CAD build for the part. Positions are in the model's coordinates, mm. A direction names the side the tool comes from. Coordinates: 2 decimals unless noted, no trailing zeros. Loops run counter-clockwise (first coordinate to the right, second up) from the corner with the lowest first, then second, coordinate; pieces in that order, holes last. Notation, with made-up numbers: (-33.75, -33) -> (22.25, -33) arc R13 cw to (22.25, -13) -> close; hole circle Ø1 at (-24, 9). An arc over 180 degrees is marked (long way). Answer as CSV lines item,"result". Start each with the question number.
```python
from build123d import *

# Parameters (mm, degrees)
SKETCH1_W               = 22.75
SKETCH1_H               = 11.15
BOSS_EXTRUDE1_DEPTH     = 19.5
SKETCH2_W               = 29.8
SKETCH2_H               = 13.8
SKETCH2_W_2             = 20.9
SKETCH2_H_2             = 8.8
BOSS_EXTRUDE2_DEPTH     = 2
FILLET1_R               = 1
BOSS_EXTRUDE3_DEPTH     = 4.5
FILLET2_R               = 1
SKETCH4_W               = 0.8
SKETCH4_H               = 6.4
BOSS_EXTRUDE4_DEPTH     = 8.7
CHAMFER1_SIZE           = 1
SKETCH5_W               = 29
SKETCH5_H               = 6.5
BOSS_EXTRUDE5_DEPTH     = 8.7
SKETCH6_W               = 22.75
SKETCH6_H               = 11.78
BOSS_EXTRUDE6_DEPTH     = 3.5
CHAMFER2_SIZE           = 0.5
CUT_EXTRUDE1_DEPTH      = 34.821116013
CUT_EXTRUDE1_DEPTH_BACK = 34.821116013
SKETCH7_R               = 0.871711707


with BuildPart() as part:
    # Sketch1 → Boss-Extrude1 (new body)
    with BuildSketch(Plane(origin=(0, 0, 0), x_dir=(1, 0, 0), z_dir=(0, 1, 0))):
        Rectangle(SKETCH1_W, SKETCH1_H)
    extrude(amount=BOSS_EXTRUDE1_DEPTH)

    # Sketch2 → Boss-Extrude2 (add)
    with BuildSketch(Plane(origin=(0, 19.5, 0), x_dir=(1, 0, 0), z_dir=(0, 1, 0))):
        Rectangle(SKETCH2_W, SKETCH2_H)
        Rectangle(SKETCH2_W_2, SKETCH2_H_2, mode=Mode.SUBTRACT)
    extrude(amount=BOSS_EXTRUDE2_DEPTH)

    # Fillet1
    fillet1_edges = [part.edges().sort_by_distance(p)[0] for p in [
        (14.9, 21.5, 0),
        (0, 21.5, -6.9),
        (-14.9, 21.5, 0),
        (0, 21.5, 6.9),
        (14.9, 20.5, 6.9),
        (14.9, 20.5, -6.9),
        (-14.9, 20.5, -6.9),
        (-14.9, 20.5, 6.9),
    ]]
    fillet(fillet1_edges, radius=FILLET1_R)

    # Sketch3 → Boss-Extrude3 (add, symmetric)
    with BuildSketch(Plane.XY):
        with BuildLine():
            ThreePointArc((-7.628944694, 29.986265243), (-9.732417399, 24.929551358), (-10.45, 19.5))
            Line((-10.45, 19.5), (10.45, 19.5))
            ThreePointArc((10.45, 19.5), (0.729024757, 23.568181114), (-7.628944694, 29.986265243))
        make_face()
    extrude(amount=BOSS_EXTRUDE3_DEPTH, both=True)

    # Fillet2
    fillet2_edges = [part.edges().sort_by_distance(p)[0] for p in [
        (-7.628944694, 29.986265243, 0),
    ]]
    fillet(fillet2_edges, radius=FILLET2_R)

    # Sketch4 → Boss-Extrude4 (add)
    with BuildSketch(Plane(origin=(0, 0, 0), x_dir=(-1, 0, 0), z_dir=(0, -1, 0))):
        with Locations((-6.375, 0)):
            Rectangle(SKETCH4_W, SKETCH4_H)
        with Locations((0.025, 0)):
            Rectangle(SKETCH4_W, SKETCH4_H)
    extrude(amount=BOSS_EXTRUDE4_DEPTH)

    # Chamfer1
    chamfer1_edges = [part.edges().sort_by_distance(p)[0] for p in [
        (6.375, -8.7, 3.2),
        (6.375, -8.7, -3.2),
        (-0.025, -8.7, 3.2),
        (-0.025, -8.7, -3.2),
    ]]
    chamfer(chamfer1_edges, length=CHAMFER1_SIZE)

    # Sketch5 → Boss-Extrude5 (add)
    with BuildSketch(Plane.XZ.offset(-19.5)):
        Rectangle(SKETCH5_W, SKETCH5_H)
    extrude(amount=BOSS_EXTRUDE5_DEPTH)

    # Sketch6 → Boss-Extrude6 (add)
    with BuildSketch(Plane.XZ.offset(-19.5)):
        Rectangle(SKETCH6_W, SKETCH6_H)
    extrude(amount=BOSS_EXTRUDE6_DEPTH)

    # Chamfer2
    # the kernel refuses this chamfer: 0.5 mm, written as the material it takes off along each edge
    with BuildSketch(Plane(origin=(-12.660841494, 16, -5.89), x_dir=(0, -0.027495876610585647, 0.9996219169112968), z_dir=(1, 0, 0))) as chamfer2_piece_1_section:
        Polygon((CHAMFER2_SIZE * 0.999621916911, -CHAMFER2_SIZE * 0.0274958766106), (-CHAMFER2_SIZE * 0.0274958766106, -CHAMFER2_SIZE * 0.999621916911), (0, 0), align=None)
    chamfer2_piece_1 = extrude(amount=25.321682988, mode=Mode.PRIVATE)
    chamfer2_piece_1 = split(chamfer2_piece_1, bisect_by=Plane(origin=(0, 16.184966798, -5.575), z_dir=(0, 0, -1)), keep=Keep.TOP, mode=Mode.PRIVATE)
    add(chamfer2_piece_1, mode=Mode.SUBTRACT)
    with BuildSketch(Plane(origin=(12.660841494, 16, 5.89), x_dir=(0, 0.9996219169112968, 0.02749587661058555), z_dir=(-1, 0, 0))) as chamfer2_piece_2_section:
        Polygon((CHAMFER2_SIZE * 0.999621916911, CHAMFER2_SIZE * 0.0274958766106), (-CHAMFER2_SIZE * 0.0274958766106, CHAMFER2_SIZE * 0.999621916911), (0, 0), align=None)
    chamfer2_piece_2 = extrude(amount=25.321682988, mode=Mode.PRIVATE)
    chamfer2_piece_2 = split(chamfer2_piece_2, bisect_by=Plane(origin=(0, 16.184966798, 5.575), z_dir=(0, 0, 1)), keep=Keep.TOP, mode=Mode.PRIVATE)
    add(chamfer2_piece_2, mode=Mode.SUBTRACT)

    # Sketch7 → Cut-Extrude1 (cut, two sides: drawn at the far end of the back side and taken through both)
    with BuildSketch(Plane.ZY.offset(0.425).offset(-CUT_EXTRUDE1_DEPTH_BACK)):
        with Locations((0, -6.204058817)):
            Circle(SKETCH7_R)
    extrude(amount=CUT_EXTRUDE1_DEPTH + CUT_EXTRUDE1_DEPTH_BACK, mode=Mode.SUBTRACT)


solid = part.part
```
Q1. Which spindle directions (+Z, -Z, +X, -X, +Y, -Y) get a long thin tool onto all of the face, cutting with end or side? Do faces 4 (the flat face through (-0.425, -4, 0)), 5 (the flat face through (13, 10.8, 0)), 6 (the flat face through (6.4, -3.8, -3.2)), 7 (the flat face through (0, 21.5, 5)). Say none if no direction does.
Q2. Two-plate mould, pull along X, no slides. Class faces 1 (the flat face through (0.375, -4, 0)), 2 (the flat face through (-14.5, 15, 0)), 3 (the flat face through (-13, 15, -3.25)): pulls with the +X half, pulls with the -X half, needs draft (parallel to the pull), parting line crosses it, or undercut.
Q3. Saw through at A-A (x = 9.25). List the corners of the cut face in (y, z) (3 decimals).
Q4. Pin check, flat tips, straight feed: pin 1 Ø0.9 at (x, y) = (6.5, -4) entering from +Z; pin 2 Ø1 at (x, y) = (-12, 4) entering from -Z; pin 3 Ø6 at (y, z) = (9, -4.5) entering from -X; pin 4 Ø4 at (y, z) = (0, 1.5) entering from +X (3 decimals). Stop position of each tip, or through.
Q5. Saw through at D-D (y = 13.5). List the corners of the cut face in (x, z) (3 decimals).
Q6. Saw through at B-B (y = 20). Give the number of separate pieces and of enclosed holes in the cut face, and give its area (3 significant figures).
Q7. Probe probe 1 along X at (y, z) = (-3, -1.75) (3 decimals); probe 2 along Z at (x, y) = (4.25, 10.5) (3 decimals); probe 3 along Y at (x, z) = (3, -6). List the from-to ranges inside material, lowest first. Write a range as from..to.
Ans:
1,face 4,"+Z, -Z, -X, -Y"
1,face 5,"+Z, -Z, +X, -Y"
1,face 6,"-Z, +X, -X, -Y"
1,face 7,"+Y"
2,face 1,"undercut"
2,face 2,"pulls with the -X half"
2,face 3,"needs draft"
3,outline,"(0, -5.575) -> (16.185, -5.575) -> (16.5, -5.89) -> (19.5, -5.89) -> (19.5, -6.9) -> (20.5, -6.9) arc R1 ccw to (21.5, -5.9) -> (21.5, -4.4) -> (19.848, -4.4) -> (19.848, 4.4) -> (21.5, 4.4) -> (21.5, 5.9) arc R1 ccw to (20.5, 6.9) -> (19.5, 6.9) -> (19.5, 5.89) -> (16.5, 5.89) -> (16.185, 5.575) -> (0, 5.575) -> close"
4,pin 1,"stops at z = 3.2"
4,pin 2,"passes through"
4,pin 3,"stops at x = -14.5"
4,pin 4,"stops at x = 11.375"
5,outline,"(-14.5, -3.25) -> (-11.375, -3.25) -> (-11.375, -5.575) -> (11.375, -5.575) -> (11.375, -3.25) -> (14.5, -3.25) -> (14.5, 3.25) -> (11.375, 3.25) -> (11.375, 5.575) -> (-11.375, 5.575) -> (-11.375, 3.25) -> (-14.5, 3.25) -> close"
6,separate pieces,"1"
6,enclosed holes,"2"
6,area,"396 mm²"
7,probe 1,"x = -0.425..0.375, 5.975..6.775"
7,probe 2,"z = -5.575..5.575"
7,probe 3,"y = 19.5..21.49"
